from build123d import *

# Parameters (mm, degrees)
F0_R     = 1.75
F1_DEPTH = 5
F3_DEPTH = 7
F5_DEPTH = 5
F6_W     = 1
F6_H     = 1
F7_DEPTH = 6
F8_W     = 1
F8_H     = 1
F9_DEPTH = 6


with BuildPart() as f1:
    # F0 (on Top) → F1 (new body)
    with BuildSketch(Plane.XY):
        with BuildLine():
            ThreePointArc((-0.9388981295, -10.4579381478), (0, 10.5), (0.9388981295, -10.4579381478))
            Line((0.9388981295, -10.4579381478), (0.9388981295, -14.9705868389))
            Line((0.9388981295, -14.9705868389), (0.9388981295, -22.7195436882))
            Line((0.9388981295, -22.7195436882), (4.4024475525, -22.7195436882))
            Line((4.4024475525, -22.7195436882), (10.116501772, -22.7195436882))
            Line((10.116501772, -22.7195436882), (21.0318053748, -18.9101754503))
            Line((21.0318053748, -18.9101754503), (21.0318053748, -15))
            Line((21.0318053748, -15), (15.0318053748, -15))
            Line((15.0318053748, -15), (15.0318053748, -14))
            Line((15.0318053748, -14), (21.0318053748, -14))
            Line((21.0318053748, -14), (21.0318053748, -9.7105238683))
            Line((21.0318053748, -9.7105238683), (11.4326605041, -9.7105238683))
            ThreePointArc((11.4326605041, -9.7105238683), (14.9816222336, -0.7422905424), (12.3365595381, 8.5328365016))
            ThreePointArc((12.3365595381, 8.5328365016), (11.704066925, 11.7858634787), (13.6674751693, 14.4555562485))
            Line((13.6674751693, 14.4555562485), (37.7463729757, 28.3575143788))
            Line((37.7463729757, 28.3575143788), (38.825355636, 26.4886615908))
            Line((38.825355636, 26.4886615908), (48.0623036168, 31.821615994))
            Line((48.0623036168, 31.821615994), (43.9043382963, 39.0234231853))
            Line((43.9043382963, 39.0234231853), (34.6673903154, 33.6904687821))
            Line((34.6673903154, 33.6904687821), (35.7463729757, 31.821615994))
            Line((35.7463729757, 31.821615994), (6.9158291977, 15.1762937829))
            ThreePointArc((6.9158291977, 15.1762937829), (5.1654246928, 14.5629294653), (3.3118718983, 14.6298156013))
            ThreePointArc((3.3118718983, 14.6298156013), (0, 15), (-3.3118718983, 14.6298156013))
            ThreePointArc((-3.3118718983, 14.6298156013), (-5.1654246928, 14.5629294653), (-6.9158291977, 15.1762937829))
            Line((-6.9158291977, 15.1762937829), (-35.7463729757, 31.821615994))
            Line((-35.7463729757, 31.821615994), (-34.6673903154, 33.6904687821))
            Line((-34.6673903154, 33.6904687821), (-43.9043382963, 39.0234231853))
            Line((-43.9043382963, 39.0234231853), (-48.0623036168, 31.821615994))
            Line((-48.0623036168, 31.821615994), (-38.825355636, 26.4886615908))
            Line((-38.825355636, 26.4886615908), (-37.7463729757, 28.3575143788))
            Line((-37.7463729757, 28.3575143788), (-18.5453659437, 17.2718078002))
            ThreePointArc((-18.5453659437, 17.2718078002), (-18.1373653852, 16.2868073185), (-18.9832044744, 15.6377721578))
            Line((-18.9832044744, 15.6377721578), (-24.1605976116, 15.6377721578))
            Line((-24.1605976116, 15.6377721578), (-24.1605976116, 10.7727729008))
            Line((-24.1605976116, 10.7727729008), (-18.1605976116, 10.7727729008))
            Line((-18.1605976116, 10.7727729008), (-18.1605976116, 9.7727729008))
            Line((-18.1605976116, 9.7727729008), (-24.1605976116, 9.7727729008))
            Line((-24.1605976116, 9.7727729008), (-24.1605976116, 6.9246333643))
            Line((-24.1605976116, 6.9246333643), (-13.3059931147, 6.9246333643))
            ThreePointArc((-13.3059931147, 6.9246333643), (-13.6917078006, -6.1267558709), (-3.7029089872, -14.5357650309))
            Line((-3.7029089872, -14.5357650309), (-3.7029089872, -22.7195436882))
            Line((-3.7029089872, -22.7195436882), (-0.9388981295, -22.7195436882))
            Line((-0.9388981295, -22.7195436882), (-0.9388981295, -14.9705868389))
            Line((-0.9388981295, -14.9705868389), (-0.9388981295, -10.4579381478))
        make_face()
        with Locations((-41.3648469661, 32.756042388)):
            Circle(F0_R, mode=Mode.SUBTRACT)
        with Locations((41.3648469661, 32.756042388)):
            Circle(F0_R, mode=Mode.SUBTRACT)
    extrude(amount=F1_DEPTH)

    # F2 (on face) → F3 (join)
    with BuildSketch(Plane.XY.offset(5)):
        with BuildLine():
            Line((37.7463729757, 28.3575143788), (35.7463729757, 31.821615994))
            Line((35.7463729757, 31.821615994), (6.9158291977, 15.1762937829))
            ThreePointArc((6.9158291977, 15.1762937829), (5.1654246928, 14.5629294653), (3.3118718983, 14.6298156013))
            ThreePointArc((3.3118718983, 14.6298156013), (0, 15), (-3.3118718983, 14.6298156013))
            ThreePointArc((-3.3118718983, 14.6298156013), (-5.1654246928, 14.5629294653), (-6.9158291977, 15.1762937829))
            Line((-6.9158291977, 15.1762937829), (-35.7463729757, 31.821615994))
            Line((-35.7463729757, 31.821615994), (-37.7463729757, 28.3575143788))
            Line((-37.7463729757, 28.3575143788), (-18.5453659437, 17.2718078002))
            ThreePointArc((-18.5453659437, 17.2718078002), (-18.1373653852, 16.2868073185), (-18.9832044744, 15.6377721578))
            Line((-18.9832044744, 15.6377721578), (-24.1605976116, 15.6377721578))
            Line((-24.1605976116, 15.6377721578), (-24.1605976116, 10.7727729008))
            Line((-24.1605976116, 10.7727729008), (-18.1605976116, 10.7727729008))
            Line((-18.1605976116, 10.7727729008), (-18.1605976116, 9.7727729008))
            Line((-18.1605976116, 9.7727729008), (-24.1605976116, 9.7727729008))
            Line((-24.1605976116, 9.7727729008), (-24.1605976116, 6.9246333643))
            Line((-24.1605976116, 6.9246333643), (-13.3059931147, 6.9246333643))
            ThreePointArc((-13.3059931147, 6.9246333643), (-13.6917078006, -6.1267558709), (-3.7029089872, -14.5357650309))
            Line((-3.7029089872, -14.5357650309), (-3.7029089872, -22.7195436882))
            Line((-3.7029089872, -22.7195436882), (-0.9388981295, -22.7195436882))
            Line((-0.9388981295, -22.7195436882), (-0.9388981295, -10.4579381478))
            ThreePointArc((-0.9388981295, -10.4579381478), (0, 10.5), (0.9388981295, -10.4579381478))
            Line((0.9388981295, -10.4579381478), (0.9388981295, -22.7195436882))
            Line((0.9388981295, -22.7195436882), (10.116501772, -22.7195436882))
            Line((10.116501772, -22.7195436882), (21.0318053748, -18.9101754503))
            Line((21.0318053748, -18.9101754503), (21.0318053748, -15))
            Line((21.0318053748, -15), (15.0318053748, -15))
            Line((15.0318053748, -15), (15.0318053748, -14))
            Line((15.0318053748, -14), (21.0318053748, -14))
            Line((21.0318053748, -14), (21.0318053748, -9.7105238683))
            Line((21.0318053748, -9.7105238683), (11.4326605041, -9.7105238683))
            ThreePointArc((11.4326605041, -9.7105238683), (14.9816222336, -0.7422905424), (12.3365595381, 8.5328365016))
            ThreePointArc((12.3365595381, 8.5328365016), (11.704066925, 11.7858634787), (13.6674751693, 14.4555562485))
            Line((13.6674751693, 14.4555562485), (37.7463729757, 28.3575143788))
        make_face()
    extrude(amount=F3_DEPTH)

    # F4 (on face) → F5 (join)
    with BuildSketch(Plane.XY.offset(12)):
        with BuildLine():
            Line((0.9388981295, -22.7195436882), (3.4428494982, -22.7195436882))
            Line((3.4428494982, -22.7195436882), (3.4428494982, -14.5995475044))
            ThreePointArc((3.4428494982, -14.5995475044), (7.8291658231, -12.7946927479), (11.4326605041, -9.7105238683))
            ThreePointArc((11.4326605041, -9.7105238683), (14.9816222336, -0.7422905424), (12.3365595381, 8.5328365016))
            ThreePointArc((12.3365595381, 8.5328365016), (11.704066925, 11.7858634787), (13.6674751693, 14.4555562485))
            Line((13.6674751693, 14.4555562485), (37.7463729757, 28.3575143788))
            Line((37.7463729757, 28.3575143788), (35.7463729757, 31.821615994))
            Line((35.7463729757, 31.821615994), (6.9158291977, 15.1762937829))
            ThreePointArc((6.9158291977, 15.1762937829), (5.1654246928, 14.5629294653), (3.3118718983, 14.6298156013))
            ThreePointArc((3.3118718983, 14.6298156013), (0, 15), (-3.3118718983, 14.6298156013))
            ThreePointArc((-3.3118718983, 14.6298156013), (-5.1654246928, 14.5629294653), (-6.9158291977, 15.1762937829))
            Line((-6.9158291977, 15.1762937829), (-35.7463729757, 31.821615994))
            Line((-35.7463729757, 31.821615994), (-37.7463729757, 28.3575143788))
            Line((-37.7463729757, 28.3575143788), (-18.5453659437, 17.2718078002))
            Line((-18.5453659437, 17.2718078002), (-11.7966768619, 13.3754503421))
            ThreePointArc((-11.7966768619, 13.3754503421), (-10.7011937418, 11.7891096419), (-11.2363395942, 9.9370353992))
            ThreePointArc((-11.2363395942, 9.9370353992), (-12.3632586806, 8.4941058856), (-13.3059931147, 6.9246333643))
            ThreePointArc((-13.3059931147, 6.9246333643), (-13.6917078006, -6.1267558709), (-3.7029089872, -14.5357650309))
            Line((-3.7029089872, -14.5357650309), (-3.7029089872, -22.7195436882))
            Line((-3.7029089872, -22.7195436882), (-0.9388981295, -22.7195436882))
            Line((-0.9388981295, -22.7195436882), (-0.9388981295, -10.4579381478))
            ThreePointArc((-0.9388981295, -10.4579381478), (0, 10.5), (0.9388981295, -10.4579381478))
            Line((0.9388981295, -10.4579381478), (0.9388981295, -22.7195436882))
        make_face()
    extrude(amount=F5_DEPTH)

    # F6 (on face) → F7 (cut)
    with BuildSketch(Plane.YZ.offset(21.0318053748)):
        with Locations((-15.5, 9.5)):
            Rectangle(F6_W, F6_H)
        with Locations((-15.5, 7.5)):
            Rectangle(F6_W, F6_H)
        with Locations((-15.5, 11.5)):
            Rectangle(F6_W, F6_H)
        with Locations((-15.5, 5.5)):
            Rectangle(F6_W, F6_H)
        with Locations((-15.5, 3.5)):
            Rectangle(F6_W, F6_H)
        with Locations((-15.5, 1.5)):
            Rectangle(F6_W, F6_H)
    extrude(amount=-F7_DEPTH, mode=Mode.SUBTRACT)

    # F8 (on face) → F9 (cut)
    with BuildSketch(Plane(origin=(-24.1605976116, 0, 0), x_dir=(0, -1, 0), z_dir=(-1, 0, 0))):
        with Locations((-11.2727729008, 11.5)):
            Rectangle(F8_W, F8_H)
        with Locations((-11.2727729008, 9.5)):
            Rectangle(F8_W, F8_H)
        with Locations((-11.2727729008, 7.5)):
            Rectangle(F8_W, F8_H)
        with Locations((-11.2727729008, 5.5)):
            Rectangle(F8_W, F8_H)
        with Locations((-11.2727729008, 3.5)):
            Rectangle(F8_W, F8_H)
        with Locations((-11.2727729008, 1.5)):
            Rectangle(F8_W, F8_H)
    extrude(amount=-F9_DEPTH, mode=Mode.SUBTRACT)


solid = f1.part
Source: CAD feature listing. Evaluate the final solid. Frame: model axes, mm. A direction names the side the tool comes from. Round coordinates to 2 decimals unless told otherwise and drop trailing zeros. Loops run counter-clockwise (first coordinate to the right, second up) from the corner with the lowest first, then second, coordinate; pieces in that order, holes last.
Q1. Section C-C, the plane y = 22.5. Return loops of the section in (x, z), plus the area to 3 significant figures.
Q2. Section B-B, the plane z = 13.75. Return loops of the section in (x, y).
Q3. Section D-D, the plane x = 0. Return loops of the section in (y, z), plus the area to 3 significant figures.
Q4. Section A-A, the plane y = -1.5. Return loops of the section in (x, z).
Q5. Mould query, pull axis Y, two halves, no side actions, for faces 5 (the face through (36.76, 30.065, 10.916)), 6 (the face through (-21, 9.773, 6)), 7 (the face through (-43.508, 29.192, 2.465)). Classes: pulls with the +Y half, pulls with the -Y half, needs draft (parallel to the pull), parting line crosses it, or undercut.
Q6. First-contact query: P1, Ø5, axis at y = -3, z = 5, coming from the +X side; P2, Ø0.5, axis at x = -20.5, z = 6.5, coming from the -Y side; P3, Ø4, axis at x = 41.36, y = 32.76, coming from the +Z side; P4, Ø5, axis at x = 8.5, y = 0, coming from the -Z side. Flat tips, straight axial feed; report the tip coordinate or a pass-through.
Q7. Access query for faces 1 (the face through (-3.703, -19, 8)), 2 (the face through (21.032, -12, 6)), 3 (the face through (-40, 31, 5)), 4 (the face through (-38.3, 27.4, 2.5)). Directions: +Z, -Z, +X, -X, +Y, -Y. A direction counts if a zero-diameter tool reaches every point of the face in a straight line with its end or side. Return the directions, or none.
Q8. Ray query, line 1 (X direction, y = 32, z = 4.75); line 2 (X direction, y = 0, z = 10.5); line 3 (X direction, y = 33, z = 2). Return the intervals inside material, ascending.
Solutions:
1. outline: (-27.6, 0) - (-19.6, 0) - (-19.6, 17) - (-27.6, 17) - close; (19.6, 0) - (27.6, 0) - (27.6, 17) - (19.6, 17) - close
1. area: 272 mm2
2. outline: (-37.75, 28.36) - (-11.8, 13.38) arc R2.25 cw to (-11.24, 9.94) arc R15 ccw to (-3.7, -14.54) - (-3.7, -22.72) - (-0.94, -22.72) - (-0.94, -10.46) arc R10.5 cw (long way) to (0.94, -10.46) - (0.94, -22.72) - (3.44, -22.72) - (3.44, -14.6) arc R15 ccw to (12.34, 8.53) arc R4.13 cw to (13.67, 14.46) - (37.75, 28.36) - (35.75, 31.82) - (6.92, 15.18) arc R5 cw to (3.31, 14.63) arc R15 ccw to (-3.31, 14.63) arc R5 cw to (-6.92, 15.18) - (-35.75, 31.82) - close
3. outline: (10.5, 0) - (15, 0) - (15, 17) - (10.5, 17) - close
3. area: 76.5 mm2
4. outline: (-14.92, 0) - (-10.39, 0) - (-10.39, 17) - (-14.92, 17) - close; (10.39, 0) - (14.92, 0) - (14.92, 17) - (10.39, 17) - close
5. face 5: pulls with the +Y half
5. face 6: undercut
5. face 7: pulls with the -Y half
6. P1: stops at x = 14.99
6. P2: stops at y = 6.92
6. P3: stops at z = 5
6. P4: stops at z = 0
7. face 1: +Z, -Z, -X, -Y
7. face 2: +Z, -Z, +X, -Y
7. face 3: +Z, -X, +Y
7. face 4: +Z, -Z, -Y
8. line 1: x = -47.96 to -42.94, -39.79 to -35.64, 35.64 to 39.79, 42.94 to 47.96
8. line 2: x = -15 to -10.5, 10.5 to 15
8. line 3: x = -47.38 to -43.1, -39.63 to -35.07, 35.07 to 39.63, 43.1 to 47.38
